CAD build for the part. Positions are in the model's coordinates, mm. Face numbers are marked on the shaded views. A direction names the side the tool comes from. Give positions to 0.01 mm unless a question says otherwise; leave off trailing zeros. Order: outer loops, then holes, each group sorted by start corner. A loop starts at its lowest first (then second) coordinate and runs counter-clockwise, first axis right, second up. Notation, with made-up numbers: M 60.5,0 L 87.5,0 A19 cw 87.5,23 Z; hole C 81,71.5 d10. An arc over 180 degrees is marked long. Put each result on its own line as item: value. Start each with the question number.
1) Cut at B-B (x = 34). Write the cut outline in (y, z), and give its area (3 significant figures).
2) Cut at A-A (z = 14.25). Write the cut outline in (x, y).
3) Pin check, flat tips, straight feed: pin 1 (1.5 mm diameter, centred on y = -14, z = 9.5, fed in from -X); pin 2 (12 mm diameter, centred on x = -14.5, y = -3, fed in from +Z); pin 3 (3 mm diameter, centred on x = -11.5, z = 3, fed in from +Y). Stop position of each tip, or through.
4) Two-plate mould, pull along Y, no slides. Class the marked faces 3, 4 and 5: released by +Y, released by -Y, zero draft, split by the parting line, or undercut.
5) Cut at C-C (y = -3.75). Write the cut outline in (x, z).
6) Drill centre lines: line 1 (Y direction, x = -30.5, z = 17.25); line 2 (X direction, y = -6.75, z = 16); line 3 (X direction, y = 12.25, z = 17.25). Where is each one in solid material? Low to high. Write a range as [from, to].
7) Cut at D-D (y = 1.25). Write the cut outline in (x, z), and give its area (3 significant figures).
8) Tool access for the marked faces 1 and 2: list every direction of +Z, -Z, +X, -X, +Y, -Y with a clear straight run to the whole face (end or side of a thin tool).
```python
from build123d import *

# Parameters (mm, degrees)
SKETCH_W     = 82
SKETCH_H     = 30
PAD_DEPTH    = 1
PAD001_DEPTH = 20
FILLET_R     = 2
FILLET001_R  = 2
CHAMFER_SIZE = 1


with BuildPart() as part:
    # Sketch → Pad (new body)
    with BuildSketch(Plane.XY):
        Rectangle(SKETCH_W, SKETCH_H)
    extrude(amount=PAD_DEPTH)

    # Sketch001 → Pad001 (new body)
    with BuildSketch(Plane.XY.offset(1)):
        Polygon((-41, 15), (-41, 2), (-38, 2), (-38, 12), (-28, 12), (-28, 15), align=None)
        Polygon((28, -12), (28, -15), (41, -15), (41, -2), (38, -2), (38, -12), align=None)
        Polygon((-41, -2), (-41, -15), (-28, -15), (-28, -12), (-38, -12), (-38, -2), align=None)
        Polygon((38, 2), (41, 2), (41, 15), (28, 15), (28, 12), (38, 12), align=None)
    extrude(amount=PAD001_DEPTH)

    # Fillet
    fillet_edges = [part.edges().sort_by_distance(p)[0] for p in [
        (41, -15, 11),
        (41, 15, 11),
        (-41, 15, 11),
    ]]
    fillet(fillet_edges, radius=FILLET_R)

    # Fillet001
    fillet001_edges = [part.edges().sort_by_distance(p)[0] for p in [
        (-41, -15, 11),
    ]]
    fillet(fillet001_edges, radius=FILLET001_R)

    # Chamfer
    chamfer_edges = [part.edges().sort_by_distance(p)[0] for p in [
        (-38, 7, 21),
        (-33, 12, 21),
        (-38, -7, 21),
        (-33, -12, 21),
        (33, -12, 21),
        (38, -7, 21),
        (38, 7, 21),
        (33, 12, 21),
    ]]
    chamfer(chamfer_edges, length=CHAMFER_SIZE)


solid = part.part
```
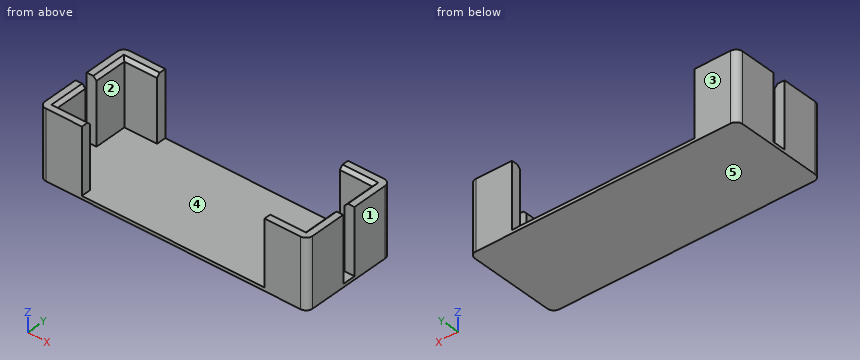
Solution:
1. outline: M -15,0 L 15,0 L 15,21 L 13,21 L 12,20 L 12,1 L -12,1 L -12,20 L -13,21 L -15,21 Z
1. area: 149 mm²
2. outline: M -41,-13 A2 ccw -39,-15 L -28,-15 L -28,-12 L -38,-12 L -38,-2 L -41,-2 Z; M -41,2 L -38,2 L -38,12 L -28,12 L -28,15 L -39,15 A2 ccw -41,13 Z; M 28,-15 L 39,-15 A2 ccw 41,-13 L 41,-2 L 38,-2 L 38,-12 L 28,-12 Z; M 28,12 L 38,12 L 38,2 L 41,2 L 41,13 A2 ccw 39,15 L 28,15 Z
3. pin 1: x = -40.98
3. pin 2: z = 1
3. pin 3: through
4. face 3: released by +Y
4. face 4: undercut
4. face 5: zero draft
5. outline: M -41,0 L 41,0 L 41,21 L 39,21 L 38,20 L 38,1 L -38,1 L -38,20 L -39,21 L -41,21 Z
6. line 1: [-15, -12], [12, 15]
6. line 2: [-41, -38], [38, 41]
6. line 3: [-41, -28], [28, 41]
7. outline: M -41,0 L 41,0 L 41,1 L -41,1 Z
7. area: 82.0 mm²
8. face 1: +Z, -Z, +X, +Y, -Y
8. face 2: +Z
